The model under review builds one solid part; all positions refer to its coordinate system, in mm. A direction names the side the tool comes from. Give positions to 0.01 mm unless a question says otherwise; leave off trailing zeros. Order: outer loops, then holes, each group sorted by start corner. A loop starts at its lowest first (then second) coordinate and runs counter-clockwise, first axis right, second up.
```python
from build123d import *

# Parameters (mm, degrees)
F3_R     = 4
F4_DEPTH = 3.9
F5_R     = 1.6
F6_DEPTH = 3.9


with BuildPart() as f1:
    # F0 (on Front) → F1 (revolve)
    with BuildSketch(Plane.XZ):
        Polygon((3.0294142647, -2.9052242924), (3.0294142647, -18.0052242924), (11.1794142647, -18.0052242924), (11.1794142647, 7.9947757076), (8.0294142647, 7.9947757076), (8.0294142647, 14.9947757076), (6.0294142647, 14.9947757076), (6.0294142647, 20.9947757076), (6.0294142647, 24.6947757076), (4.0294142647, 24.6947757076), (4.0294142647, 18.1947757076), (2.1294142647, 17.1845277874), (2.1294142647, -2.3644497353), align=None)
    revolve(axis=Axis((0.0294142647, 0, 3.3447757076), (0, 0, -1)))

    # F3 (on offset) → F4 (join)
    with BuildSketch(Plane.XY.offset(20.9947757076)):
        with BuildLine():
            ThreePointArc((-11.541230437, 4.9), (-12.7711105295, 4.4771477286), (-13.4809330315, 3.387394958))
            ThreePointArc((-13.4809330315, 3.387394958), (-13.9, 0), (-13.4809330315, -3.387394958))
            ThreePointArc((-13.4809330315, -3.387394958), (-12.7711105295, -4.4771477286), (-11.541230437, -4.9))
            Line((-11.541230437, -4.9), (11.541230437, -4.9))
            ThreePointArc((11.541230437, -4.9), (12.7711105295, -4.4771477286), (13.4809330315, -3.387394958))
            ThreePointArc((13.4809330315, -3.387394958), (13.9, 0), (13.4809330315, 3.387394958))
            ThreePointArc((13.4809330315, 3.387394958), (12.7711105295, 4.4771477286), (11.541230437, 4.9))
            Line((11.541230437, 4.9), (-11.541230437, 4.9))
        make_face()
        with Locations((0.0294142647, 0)):
            Circle(F3_R, mode=Mode.SUBTRACT)
    extrude(amount=-F4_DEPTH)

    # F5 (on face) → F6 (cut, through all)
    with BuildSketch(Plane.XY.offset(20.9947757076)):
        with Locations((-10.5, 0)):
            Circle(F5_R)
        with Locations((10.5, 0)):
            Circle(F5_R)
    extrude(amount=-F6_DEPTH, mode=Mode.SUBTRACT)


solid = f1.part
```
1. Take a section at B-B (x = -10.5). Write out the cut boundary in (y, z), and give its area (3 significant figures).
2. Take a section at D-D (z = 6.5). Write out the cut boundary in (x, y).
3. For faces 5 (the cylindrical face through (10.665, -3.349, -4.823)), 6 (the cylindrical face through (-12.1, 0.07, 19.07)), 7 (the flat face through (7, -4.9, 19)), list the 3-axis set-ups (+Z, -Z, +X, -X, +Y, -Y) from which the entire face can be reached by the end or side of a thin tool; tool diameter is ignored.
4. Insertion check: pin 1 (4 mm diameter, centred on x = 10.5, y = 0, fed in from +Z); pin 2 (4.5 mm diameter, centred on x = -6, z = 20, fed in from -Y); pin 3 (1.5 mm diameter, centred on x = 8.5, z = -2, fed in from +Y); pin 4 (2.5 mm diameter, centred on x = 0.03, y = 0, fed in from +Z). Each pin has a flat end and moves straight along its axis. Give the tip position at first contact, or say it passes through.
5. Take a section at A-A (z = 20). Write out the cut boundary in (x, y), and give its area (3 significant figures).
6. To check wall thickness, follow line 1 (X direction, y = 0, z = 11.75); line 2 (Z direction, x = -9, y = -1.5); line 3 (X direction, y = 0, z = -10.75). State the ranges of each line that lie inside material, in increasing order.
7. Take a section at C-C (y = -7). Write out the cut boundary in (x, z).
8. Draft analysis for pull direction X (two halves, no side actions). For faces 1 (the cylindrical face through (12.756, -4.488, 19.072)), 2 (the cylindrical face through (-2.35, 1.83, -10.56)), 3 (the cylindrical face through (-0.244, -2.082, 7.273)), 4 (the flat face through (3, -5.4, 14.995)), state which applies: pulls with the +X half, pulls with the -X half, needs draft (parallel to the pull), parting line crosses it, or undercut.
Answer:
1. outline: (-4.9, 17.09) - (-1.6, 17.09) - (-1.6, 20.99) - (-4.9, 20.99) - close; (-3.67, -18.01) - (3.67, -18.01) - (3.67, 7.99) - (-3.67, 7.99) - close; (1.6, 17.09) - (4.9, 17.09) - (4.9, 20.99) - (1.6, 20.99) - close
1. area: 216 mm2
2. outline: circle Ø22.3 at (0.03, 0); hole circle Ø4.2 at (0.03, 0)
3. face 5: -Z
3. face 6: +Z
3. face 7: +Z, +X, -Y
4. pin 1: stops at z = 20.99
4. pin 2: stops at y = -4.9
4. pin 3: stops at y = 8.04
4. pin 4: passes through
5. outline: (-13.48, -3.39) arc R2 ccw to (-11.54, -4.9) - (-3.43, -4.9) arc R6 ccw to (3.49, -4.9) - (11.54, -4.9) arc R2 ccw to (13.48, -3.39) arc R13.9 ccw to (13.48, 3.39) arc R2 ccw to (11.54, 4.9) - (3.49, 4.9) arc R6 ccw to (-3.43, 4.9) - (-11.54, 4.9) arc R2 ccw to (-13.48, 3.39) arc R13.9 ccw to start; hole circle Ø3.2 at (-10.5, 0); hole circle Ø8 at (0.03, 0); hole circle Ø3.2 at (10.5, 0)
5. area: 209 mm2
6. line 1: x = -7.97 to -2.07, 2.13 to 8.03
6. line 2: z = -18.01 to 7.99, 17.09 to 20.99
6. line 3: x = -11.12 to -2.97, 3.03 to 11.18
7. outline: (-8.65, -18.01) - (8.71, -18.01) - (8.71, 7.99) - (3.9, 7.99) - (3.9, 14.99) - (-3.84, 14.99) - (-3.84, 7.99) - (-8.65, 7.99) - close
8. face 1: pulls with the +X half
8. face 2: undercut
8. face 3: undercut
8. face 4: needs draft
